Work out the finished part from the listing and answer in its coordinate system (mm). A direction names the side the tool comes from. Coordinates: 2 decimals unless noted, no trailing zeros. Order: outer loops, then holes, each group sorted by start corner. A loop starts at its lowest first (then second) coordinate and runs counter-clockwise, first axis right, second up. Notation, with made-up numbers: M -16.5,58 L 34.5,58 A23 cw 34.5,86 Z; hole C 22,18.25 d4. An arc over 180 degrees is marked long. Write item = value, one per line. Start each with the question number.
Q1. Find section C-C on z = 1.3. Give the number of separate pieces and of enclosed holes in the cut face, and give its area (3 significant figures).
Q2. Find section D-D on x = 19. Give the vertices of the cut face in (y, z) (3 decimals), and give its area (3 significant figures).
Q3. Determine the mould class of faces 1 (the flat face through (-79.5, 0, 2)), 2 (the cylindrical face through (54.326, -6.043, 1.61)), 3 (the flat face through (-10, 22, 2)), 4 (the flat face through (-65, -20, 2)) for opening direction X: released by +X, released by -X, zero draft, split by the parting line, or undercut.
Q4. Find section B-B on x = -28.5. Give the vertices of the cut face in (y, z) (3 decimals), and give its area (3 significant figures).
Q5. Find section A-A on x = 0. Give the vertices of the cut face in (y, z) (3 decimals), and give its area (3 significant figures).
Q6. Each of these flat-tipped pins is pushed along its axis until it touches: P1, Ø1, axis at y = -21.5, z = 1, coming from the -X side; P2, Ø2, axis at x = 55, y = -2, coming from the +Z side; P3, Ø1.6, axis at x = -62, z = 1, coming from the -Y side; P4, Ø1.6, axis at y = -21.5, z = 1.5, coming from the +X side. Where does it stop, or does it pass through?
Q7. Straight lines are drawn through the part: line 1 along X through (y, z) = (-12, 1.05); line 2 along X through (y, z) = (-4.5, 2.45); line 3 along X through (y, z) = (3.5, 1.45). For each, find the intervals that lie inside material, in ascending order.
Q8. A tool of negligible diameter and unlimited length cuts with its end or side. For faces 5 (the flat face through (-28, -9, 2)), 6 (the flat face through (50, 22, 2)), 7 (the flat face through (-20, -20, 2)), from which of +Z, -Z, +X, -X, +Y, -Y can it reach the whole face along a straight path? Write none if from no direction.
```python
from build123d import *

# Parameters (mm, degrees)
ESQUISSE1_W             = 165.35
ESQUISSE1_H             = 46.35
BOSS_EXTRU_1_DEPTH      = 3.175
ESQUISSE5_W             = 20
ESQUISSE5_H             = 3.175
ESQUISSE5_W_2           = 26.325
ENL_V_MAT_EXTRU_2_DEPTH = 86.920410119
ESQUISSE7_W             = 3.175
ESQUISSE7_H             = 46.35
ENL_V_MAT_EXTRU_4_DEPTH = 86.920410119
ESQUISSE8_W             = 3.175
ESQUISSE8_H             = 3.175
ENL_V_MAT_EXTRU_5_DEPTH = 83.869845239
ESQUISSE6_R             = 8
ENL_V_MAT_EXTRU_3_DEPTH = 83.869845239
ESQUISSE9_W             = 40
ESQUISSE9_H             = 8
ENL_V_MAT_EXTRU_6_DEPTH = 83.869845239
CONG_1_R                = 3


with BuildPart() as part:
    # Esquisse1 → Boss.-Extru.1 (new body)
    with BuildSketch(Plane.XY):
        Rectangle(ESQUISSE1_W, ESQUISSE1_H)
    extrude(amount=BOSS_EXTRU_1_DEPTH)

    # Esquisse5 → Enlèv. mat.-Extru.2 (cut, through all)
    with BuildSketch(Plane.XY.offset(3.175)):
        with Locations((-20, -21.5875)):
            Rectangle(ESQUISSE5_W, ESQUISSE5_H)
        with Locations((20, -21.5875)):
            Rectangle(ESQUISSE5_W, ESQUISSE5_H)
        with Locations((63.1625, -21.5875)):
            Rectangle(ESQUISSE5_W_2, ESQUISSE5_H)
        with Locations((-63.1625, -21.5875)):
            Rectangle(ESQUISSE5_W_2, ESQUISSE5_H)
    enl_v_mat_extru_2 = extrude(amount=-ENL_V_MAT_EXTRU_2_DEPTH, mode=Mode.SUBTRACT)

    # Symétrie2: Enlèv. mat.-Extru.2 across plane
    add(enl_v_mat_extru_2.mirror(Plane.ZX), mode=Mode.SUBTRACT)

    # Esquisse7 → Enlèv. mat.-Extru.4 (cut, through all)
    with BuildSketch(Plane.XY.offset(3.175)):
        with Locations((-81.0875, 0)):
            Rectangle(ESQUISSE7_W, ESQUISSE7_H)
        with Locations((81.0875, 0)):
            Rectangle(ESQUISSE7_W, ESQUISSE7_H)
    extrude(amount=-ENL_V_MAT_EXTRU_4_DEPTH, mode=Mode.SUBTRACT)

    # Esquisse8 → Enlèv. mat.-Extru.5 (cut, through all)
    with BuildSketch(Plane.XY.offset(3.175)):
        with Locations((-77.9125, 21.5875)):
            Rectangle(ESQUISSE8_W, ESQUISSE8_H)
        with Locations((-77.9125, -21.5875)):
            Rectangle(ESQUISSE8_W, ESQUISSE8_H)
        with Locations((77.9125, -21.5875)):
            Rectangle(ESQUISSE8_W, ESQUISSE8_H)
        with Locations((77.9125, 21.5875)):
            Rectangle(ESQUISSE8_W, ESQUISSE8_H)
    extrude(amount=-ENL_V_MAT_EXTRU_5_DEPTH, mode=Mode.SUBTRACT)

    # Esquisse6 → Enlèv. mat.-Extru.3 (cut, through all)
    with BuildSketch(Plane.XY.offset(3.175)):
        Circle(ESQUISSE6_R)
        with Locations((60.675, -1.175)):
            Circle(ESQUISSE6_R)
    extrude(amount=-ENL_V_MAT_EXTRU_3_DEPTH, mode=Mode.SUBTRACT)

    # Esquisse9 → Enlèv. mat.-Extru.6 (cut, through all)
    with BuildSketch(Plane.XY.offset(3.175)):
        with Locations((-28, -13)):
            Rectangle(ESQUISSE9_W, ESQUISSE9_H)
    extrude(amount=-ENL_V_MAT_EXTRU_6_DEPTH, mode=Mode.SUBTRACT)

    # Congé1
    cong_1_edges = [part.edges().sort_by_distance(p)[0] for p in [
        (-48, -17, 1.5875),
        (-48, -9, 1.5875),
        (-8, -9, 1.5875),
        (-8, -17, 1.5875),
    ]]
    fillet(cong_1_edges, radius=CONG_1_R)


solid = part.part
```
Findings below:
q1.separate_pieces = 1
q1.enclosed_holes = 3
q1.area = 6,030 mm^2
q2.outline = M -20,0 L 20,0 L 20,3.175 L -20,3.175 Z
q2.area = 127 mm^2
q3.face_1 = released by -X
q3.face_2 = undercut
q3.face_3 = undercut
q3.face_4 = zero draft
q4.outline = M -20,0 L -17,0 L -17,3.175 L -20,3.175 Z; M -9,0 L 20,0 L 20,3.175 L -9,3.175 Z
q4.area = 102 mm^2
q5.outline = M -23.175,0 L -8,0 L -8,3.175 L -23.175,3.175 Z; M 8,0 L 23.175,0 L 23.175,3.175 L 8,3.175 Z
q5.area = 96.4 mm^2
q6.P1 = -50
q6.P2 = through
q6.P3 = -20
q6.P4 = 50
q7.line_1 = -79.5 to -48, -8 to 79.5
q7.line_2 = -79.5 to -6.61, 6.61 to 53.4, 67.95 to 79.5
q7.line_3 = -79.5 to -7.19, 7.19 to 54.18, 67.17 to 79.5
q8.face_5 = +Z, -Z
q8.face_6 = +Z, -Z, +X, +Y
q8.face_7 = +Z, -Z, -Y
